```python
from build123d import *

# Parameters (mm, degrees)
F0_W      = 101.6
F0_H      = 50.8
F1_DEPTH  = 19.05
F2_W      = 88.9
F2_H      = 6.35
F3_DEPTH  = 12.7
F4_W      = 76.2
F4_H      = 38.1
F5_DEPTH  = 12.7
F6_W      = 25.4
F6_H      = 10.16
F7_DEPTH  = 25.4
F8_W      = 19.9136
F8_H      = 12.7
F9_DEPTH  = 6.35
F10_W     = 12.7
F10_H     = 12.7
F11_DEPTH = 63.5
F12_W     = 12.7
F12_H     = 12.7
F13_DEPTH = 6.35
F15_DEPTH = 101.6
F16_W     = 2.794
F16_H     = 2.794
F17_DEPTH = 6.35
F18_W     = 0.508
F18_H     = 1.235321
F19_DEPTH = 2.54


with BuildPart() as f1:
    # F0 (on Top) → F1 (new body)
    with BuildSketch(Plane.XY):
        with Locations((7.125289, -7.990768)):
            Rectangle(F0_W, F0_H)
    extrude(amount=F1_DEPTH)

    # F2 (on face) → F3 (cut)
    with BuildSketch(Plane.XY.offset(19.05)):
        Polygon((-37.324711, -27.040768), (-37.324711, 17.409232), (-43.674711, 17.409232), (-43.674711, -33.390768), (-37.324711, -33.390768), align=None)
        with Locations((7.125289, -30.215768)):
            Rectangle(F2_W, F2_H)
        Polygon((57.925289, 17.409232), (51.575289, 17.409232), (51.575289, -27.040768), (51.575289, -33.390768), (57.925289, -33.390768), align=None)
    extrude(amount=-F3_DEPTH, mode=Mode.SUBTRACT)

    # F4 (on face) → F5 (cut)
    with BuildSketch(Plane(origin=(0, 0, 0), x_dir=(1, 0, 0), z_dir=(0, 0, -1))):
        with Locations((7.125289, 1.640768)):
            Rectangle(F4_W, F4_H)
    extrude(amount=-F5_DEPTH, mode=Mode.SUBTRACT)

    # F6 (on face) → F7 (cut)
    with BuildSketch(Plane(origin=(0, 0, 12.7), x_dir=(1, 0, 0), z_dir=(0, 0, -1))):
        with Locations((7.125289, 15.610768)):
            Rectangle(F6_W, F6_H)
    extrude(amount=-F7_DEPTH, mode=Mode.SUBTRACT)

    # F8 (on face) → F9 (cut)
    with BuildSketch(Plane(origin=(0, 0, 0), x_dir=(1, 0, 0), z_dir=(0, 0, -1))):
        with Locations((7.125289, 27.040768)):
            Rectangle(F8_W, F8_H)
    extrude(amount=-F9_DEPTH, mode=Mode.SUBTRACT)

    # F10 (on face) → F11 (join)
    with BuildSketch(Plane(origin=(0, 0, 0), x_dir=(1, 0, 0), z_dir=(0, 0, -1))):
        with Locations((23.432089, 27.040768)):
            Rectangle(F10_W, F10_H)
        with Locations((-9.181511, 27.040768)):
            Rectangle(F10_W, F10_H)
    extrude(amount=F11_DEPTH)

    # F12 (on face) → F13 (join)
    with BuildSketch(Plane(origin=(0, 0, -63.5), x_dir=(1, 0, 0), z_dir=(0, 0, -1))):
        Polygon((-43.674711, 33.390768), (-43.674711, -42.809232), (57.925289, -42.809232), (57.925289, 33.390768), (-2.831511, 33.390768), (-2.831511, 20.690768), (-15.531511, 20.690768), (-15.531511, 33.390768), align=None)
        with Locations((-9.181511, 27.040768)):
            Rectangle(F12_W, F12_H)
    extrude(amount=F13_DEPTH)

    # F14 (on face) → F15 (cut)
    with BuildSketch(Plane.YZ.offset(57.925289)):
        Polygon((38.046732, -63.5), (42.809232, -69.85), (42.809232, -63.5), align=None)
    extrude(amount=-F15_DEPTH, mode=Mode.SUBTRACT)

    # F16 (on face) → F17 (join)
    with BuildSketch(Plane.XY.offset(6.35)):
        with Locations((-40.499711, -3.799768)):
            Rectangle(F16_W, F16_H)
        with Locations((-40.499711, -19.293768)):
            Rectangle(F16_W, F16_H)
        with Locations((54.750289, -3.799768)):
            Rectangle(F16_W, F16_H)
        with Locations((54.750289, -19.293768)):
            Rectangle(F16_W, F16_H)
    extrude(amount=F17_DEPTH)

    # F18 (on face) → F19 (join)
    with BuildSketch(Plane.XZ.offset(33.390768)):
        Polygon((10.681289, -67.564), (10.681289, -68.326), (12.205289, -68.326), (12.205289, -65.024), (10.681289, -65.024), (10.681289, -65.786), (11.443289, -65.786), (11.443289, -67.564), align=None)
        Polygon((8.395289, -68.326), (9.919289, -68.326), (9.919289, -65.024), (8.395289, -65.024), (8.395289, -65.786), (9.157289, -65.786), (9.157289, -66.294), (8.649289, -66.294), (8.649289, -67.056), (9.157289, -67.056), (9.157289, -67.564), (8.395289, -67.564), align=None)
        Polygon((6.109289, -67.529321), (6.109289, -68.291321), (7.633289, -68.291321), (7.633289, -66.294), (6.871289, -66.294), (6.871289, -65.786), (7.633289, -65.786), (7.633289, -65.024), (6.109289, -65.024), (6.109289, -67.021321), (6.871289, -67.021321), (6.871289, -67.529321), align=None)
        Polygon((3.823289, -68.291321), (5.347289, -68.291321), (5.347289, -65.024), (4.839289, -65.024), (4.839289, -66.04), (4.331289, -66.04), (4.331289, -65.024), (3.823289, -65.024), align=None)
        with Locations((4.585289, -67.165661)):
            Rectangle(F18_W, F18_H, mode=Mode.SUBTRACT)
        Polygon((2.299289, -68.291321), (3.061289, -68.291321), (3.061289, -65.024), (2.680289, -65.024), (2.680289, -65.786), (2.299289, -65.786), (1.918289, -65.42404), (1.918289, -65.024), (1.537289, -65.024), (1.537289, -65.42404), (1.918289, -65.786), (1.537289, -66.187042), (1.537289, -67.823172), (1.918289, -68.291321), align=None)
        Polygon((2.108789, -66.187042), (2.680289, -66.187042), (2.680289, -67.823172), (2.108789, -67.823172), (1.918289, -67.642192), (1.918289, -66.387562), align=None, mode=Mode.SUBTRACT)
    extrude(amount=F19_DEPTH)


solid = f1.part
```
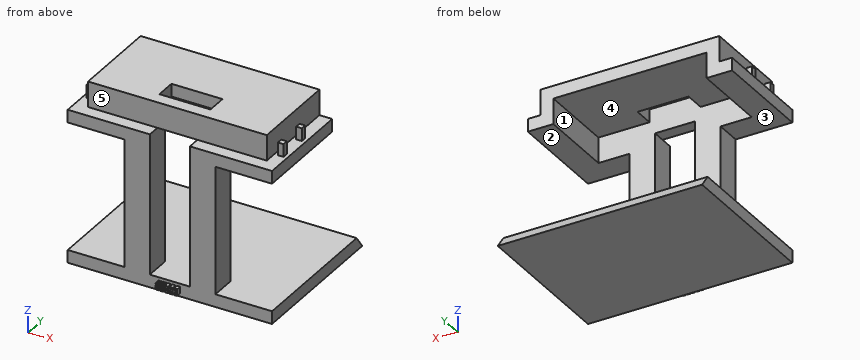
Geometry: final body of the model. Coordinates: model frame, mm. Face numbers are marked on the shaded views. A direction names the side the tool comes from. Coordinates: 2 decimals unless noted, no trailing zeros. Order: outer loops, then holes, each group sorted by start corner. A loop starts at its lowest first (then second) coordinate and runs counter-clockwise, first axis right, second up. Notation, with made-up numbers: (-8.5, 18) -> (6.5, 18) arc R20 ccw to (6.5, 38) -> close; hole circle Ø5 at (17, -27.5). An arc over 180 degrees is marked (long way). Write item = value, one per line.
(1) Pull-direction query (X, two-part tool) for the marked faces 4 and 5; classes: pulls with the +X half, pulls with the -X half, needs draft (parallel to the pull), parting line crosses it, or undercut.
Solved:
face_4 = undercut
face_5 = needs draft
(2) Access query for the marked faces 1, 2 and 3. Directions: +Z, -Z, +X, -X, +Y, -Y. A direction counts if a zero-diameter tool reaches every point of the face in a straight line with its end or side. Return the directions, or none.
Solved:
face_1 = +Y
face_2 = +X, +Y, -Y
face_3 = -X, +Y, -Y
(3) Line query: line 1 (X direction, y = -26, z = -17); line 2 (Z direction, x = 52, y = 14.5); line 3 (Z direction, x = -24.5, y = -8). Output: solid intervals per line, ascending.
Solved:
line_1 = -15.53 to -2.83, 17.08 to 29.78
line_2 = -69.85 to -63.5, 0 to 6.35
line_3 = -69.85 to -63.5, 12.7 to 19.05
(4) Cut plane B-B on y = 9.5. Return loops of the section in (x, z).
Solved:
outline = (-43.67, -69.85) -> (57.93, -69.85) -> (57.93, -63.5) -> (-43.67, -63.5) -> close; (-43.67, 0) -> (-30.97, 0) -> (-30.97, 12.7) -> (45.23, 12.7) -> (45.23, 0) -> (57.93, 0) -> (57.93, 6.35) -> (51.58, 6.35) -> (51.58, 19.05) -> (-37.32, 19.05) -> (-37.32, 6.35) -> (-43.67, 6.35) -> close
(5) Cut plane D-D on x = 23.5. Return loops of the section in (y, z), plus the area to 3 significant figures.
Solved:
outline = (-33.39, -69.85) -> (42.81, -69.85) -> (38.05, -63.5) -> (-20.69, -63.5) -> (-20.69, 12.7) -> (17.41, 12.7) -> (17.41, 19.05) -> (-27.04, 19.05) -> (-27.04, 6.35) -> (-33.39, 6.35) -> close
area = 1,680 mm²
(6) Cut plane A-A on x = -33. Return loops of the section in (y, z).
Solved:
outline = (-33.39, -69.85) -> (42.81, -69.85) -> (38.05, -63.5) -> (-33.39, -63.5) -> close; (-33.39, 0) -> (17.41, 0) -> (17.41, 19.05) -> (-27.04, 19.05) -> (-27.04, 6.35) -> (-33.39, 6.35) -> close
(7) Pin query (flat end, axial travel): pin 1 Ø1.3 at (x, y) = (3, -34.5) entering from -Z; pin 2 Ø2 at (x, y) = (-40, -19) entering from +Z; pin 3 Ø0.6 at (y, z) = (-35, -68) entering from -X; pin 4 Ø5 at (y, z) = (12, -3.5) entering from +X. Return the tip coordinate at first contact, or that it passes through.
Solved:
pin_1 = -68.29
pin_2 = 12.7
pin_3 = 1.54
pin_4 = through
(8) Cut plane C-C on z = -14. Return loops of the section in (x, y).
Solved:
outline = (-15.53, -33.39) -> (-2.83, -33.39) -> (-2.83, -20.69) -> (-15.53, -20.69) -> close; (17.08, -33.39) -> (29.78, -33.39) -> (29.78, -20.69) -> (17.08, -20.69) -> close
